Check sheet for the modelled part. Datum: model origin and axes. Units: mm. Round coordinates to 2 decimals unless told otherwise and drop trailing zeros. Write each loop counter-clockwise with the first axis right and the second up, starting at its lowest first coordinate (ties: lowest second). Pieces come first, ordered by that corner, then holes. Notation, with made-up numbers: (68, -17) -> (93, -17) arc R19 cw to (93, 14) -> close; hole circle Ø6 at (85.25, 61). An arc over 180 degrees is marked (long way). Answer as a JSON object with one key per item and string values. Group by question number.
```python
from build123d import *

# Parameters (mm, degrees)
SKETCH1_R           = 5
BOSS_EXTRUDE1_DEPTH = 1.5


with BuildPart() as part:
    # Sketch1 → Boss-Extrude1 (new, symmetric)
    with BuildSketch(Plane.XY):
        with BuildLine():
            Line((-86.14130577, 86.468523976), (9.245091692, 11.812208921))
            ThreePointArc((9.245091692, 11.812208921), (11.812208921, -9.245091692), (-9.245091692, -11.812208921))
            Line((-9.245091692, -11.812208921), (-104.631489155, 62.844106133))
            ThreePointArc((-104.631489155, 62.844106133), (-107.198606384, 83.901406746), (-86.14130577, 86.468523976))
        make_face()
        with Locations((-95.386397462, 74.656315054)):
            Circle(SKETCH1_R, mode=Mode.SUBTRACT)
    extrude(amount=BOSS_EXTRUDE1_DEPTH, both=True)


solid = part.part
```
(1) Go/stop test with a flat-tipped pin: pin 1 Ø1 at (y, z) = (58.5, 1) entering from +X. Record where the tip stops, or that it passes through.
(2) Section check D-D on x = -78.5. Record the cut outline in (y, z), then the cut area to 3 significant figures.
(3) Section check A-A on x = -97.5. Record the cut outline in (y, z).
(4) Section check C-C on y = 8. Record the cut outline in (x, z).
(5) Scan lines: line 1 along X through (y, z) = (75.5, -0.5); line 2 along Y through (x, z) = (-91.5, 0.95); line 3 along Y through (x, z) = (-99.5, -0.8). Record each from-to range of solid material in increasing order.
(6) Release check for a two-part mould opening along Y. For faces 1 (the cylindrical face through (-90.617, 76.158, -0.021)), 2 (the cylindrical face through (-107.4, 83.64, 0.02)), 3 (the flat face through (-39.116, 49.663, 0.021)), 4 (the flat face through (-47, 38, 1.5)) record: pulls with the +Y half, pulls with the -Y half, needs draft (parallel to the pull), parting line crosses it, or undercut.
(7) Section check B-B on z = -0.5. Record the cut outline in (x, y), then the cut area to 3 significant figures.
Data:
{
 "1": {"pin 1": "stops at x = -49.77"},
 "2": {"outline": "(42.39, -1.5) -> (80.49, -1.5) -> (80.49, 1.5) -> (42.39, 1.5) -> close", "area": "114 mm²"},
 "3": {"outline": "(57.26, -1.5) -> (70.13, -1.5) -> (70.13, 1.5) -> (57.26, 1.5) -> close; (79.19, -1.5) -> (89.51, -1.5) -> (89.51, 1.5) -> (79.19, 1.5) -> close"},
 "4": {"outline": "(-34.56, -1.5) -> (12.69, -1.5) -> (12.69, 1.5) -> (-34.56, 1.5) -> close"},
 "5": {"line 1": "x = -110.36 to -100.31, -90.46 to -72.13", "line 2": "y = 52.57 to 71.51, 77.8 to 89.14", "line 3": "y = 58.83 to 71.81, 77.5 to 89.08"},
 "6": {"face 1": "undercut", "face 2": "parting line crosses it", "face 3": "pulls with the +Y half", "face 4": "needs draft"},
 "7": {"outline": "(-104.63, 62.84) -> (-9.25, -11.81) arc R15 ccw to (9.25, 11.81) -> (-86.14, 86.47) arc R15 ccw to start; hole circle Ø10 at (-95.39, 74.66)", "area": "4,260 mm²"}
}
